```python
from build123d import *

# Parameters (mm, degrees)
F0_R     = 2.6
F1_DEPTH = 2
F2_R     = 2
F3_DEPTH = 25


with BuildPart() as f1:
    # F0 (on Front) → F1 (new body)
    with BuildSketch(Plane.XZ):
        with BuildLine():
            ThreePointArc((-35.5, 0), (0, -35.5), (35.5, 0))
            ThreePointArc((35.5, 0), (0, 35.5), (-35.5, 0))
        make_face()
        with BuildLine():
            ThreePointArc((-18.1, 0), (-20.7, -2.6), (-23.3, 0))
            ThreePointArc((-23.3, 0), (-20.7, 2.6), (-18.1, 0))
        make_face(mode=Mode.SUBTRACT)
        with Locations((20.7, 0)):
            Circle(F0_R, mode=Mode.SUBTRACT)
    extrude(amount=F1_DEPTH)

    # F2 (on face) → F3 (cut)
    with BuildSketch(Plane(origin=(0, 0, 0), x_dir=(-1, 0, 0), z_dir=(0, 1, 0))):
        Circle(F2_R)
        with Locations((0, 7)):
            Circle(F2_R)
        with Locations((0, 14)):
            Circle(F2_R)
        with Locations((0, 21)):
            Circle(F2_R)
        with Locations((0, 28)):
            Circle(F2_R)
        with Locations((7, 0)):
            Circle(F2_R)
        with Locations((7, 7)):
            Circle(F2_R)
        with Locations((7, 14)):
            Circle(F2_R)
        with Locations((7, 21)):
            Circle(F2_R)
        with Locations((7, 28)):
            Circle(F2_R)
        with Locations((14, 0)):
            Circle(F2_R)
        with Locations((14, 7)):
            Circle(F2_R)
        with Locations((14, 14)):
            Circle(F2_R)
        with Locations((14, 21)):
            Circle(F2_R)
        with Locations((14, 28)):
            Circle(F2_R)
        with Locations((21, 7)):
            Circle(F2_R)
        with Locations((21, 14)):
            Circle(F2_R)
        with Locations((21, 21)):
            Circle(F2_R)
        with Locations((28, 0)):
            Circle(F2_R)
        with Locations((28, 7)):
            Circle(F2_R)
        with Locations((28, 14)):
            Circle(F2_R)
        with Locations((-7, 28)):
            Circle(F2_R)
        with Locations((-7, 21)):
            Circle(F2_R)
        with Locations((-7, 14)):
            Circle(F2_R)
        with Locations((-7, 7)):
            Circle(F2_R)
        with Locations((-7, 0)):
            Circle(F2_R)
        with Locations((-14, 28)):
            Circle(F2_R)
        with Locations((-14, 21)):
            Circle(F2_R)
        with Locations((-14, 14)):
            Circle(F2_R)
        with Locations((-14, 7)):
            Circle(F2_R)
        with Locations((-14, 0)):
            Circle(F2_R)
        with Locations((-21, 21)):
            Circle(F2_R)
        with Locations((-21, 14)):
            Circle(F2_R)
        with Locations((-21, 7)):
            Circle(F2_R)
        with Locations((-28, 14)):
            Circle(F2_R)
        with Locations((-28, 7)):
            Circle(F2_R)
        with Locations((-28, 0)):
            Circle(F2_R)
        with Locations((-28, -7)):
            Circle(F2_R)
        with Locations((-21, -7)):
            Circle(F2_R)
        with Locations((-14, -7)):
            Circle(F2_R)
        with Locations((28, -7)):
            Circle(F2_R)
        with Locations((21, -7)):
            Circle(F2_R)
        with Locations((14, -7)):
            Circle(F2_R)
        with Locations((7, -7)):
            Circle(F2_R)
        with Locations((0, -7)):
            Circle(F2_R)
        with Locations((-7, -7)):
            Circle(F2_R)
        with Locations((-28, -14)):
            Circle(F2_R)
        with Locations((-21, -14)):
            Circle(F2_R)
        with Locations((-14, -14)):
            Circle(F2_R)
        with Locations((28, -14)):
            Circle(F2_R)
        with Locations((21, -14)):
            Circle(F2_R)
        with Locations((14, -14)):
            Circle(F2_R)
        with Locations((7, -14)):
            Circle(F2_R)
        with Locations((0, -14)):
            Circle(F2_R)
        with Locations((-7, -14)):
            Circle(F2_R)
        with Locations((-21, -21)):
            Circle(F2_R)
        with Locations((-14, -21)):
            Circle(F2_R)
        with Locations((21, -21)):
            Circle(F2_R)
        with Locations((14, -21)):
            Circle(F2_R)
        with Locations((7, -21)):
            Circle(F2_R)
        with Locations((0, -21)):
            Circle(F2_R)
        with Locations((-7, -21)):
            Circle(F2_R)
        with Locations((-14, -28)):
            Circle(F2_R)
        with Locations((14, -28)):
            Circle(F2_R)
        with Locations((7, -28)):
            Circle(F2_R)
        with Locations((0, -28)):
            Circle(F2_R)
        with Locations((-7, -28)):
            Circle(F2_R)
    extrude(amount=-F3_DEPTH, mode=Mode.SUBTRACT)


solid = f1.part
```
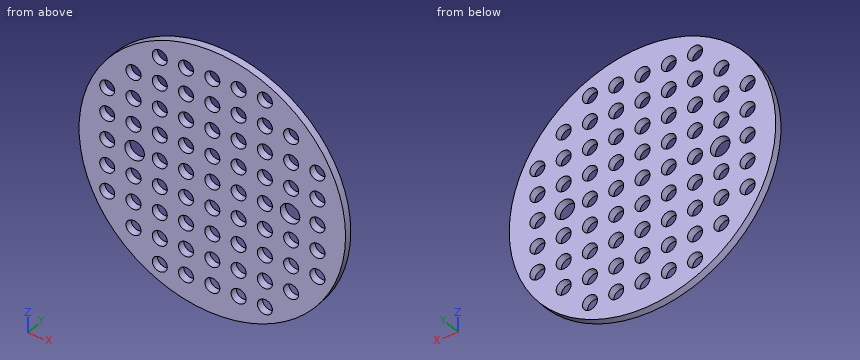
Here's how the part is built. I have some questions about the finished solid (model axes, mm). Round coordinates to 2 decimals unless told otherwise and drop trailing zeros.
1. Suppose I cut it at A-A, the plane x = 0. Give the number of separate pieces and of enclosed holes in the cut face, and give its area (3 significant figures).
Answers:
separate pieces: 10
enclosed holes: 0
area: 70.0 mm2
2. If I drill on probe 1 along Z at (x, y) = (28, -0.55); probe 2 along Z at (x, y) = (2.5, -1.8); probe 3 along X at (y, z) = (-1.15, 3.5), over which ranges is the centre line in solid material (lowest first)?
Answers:
probe 1: z = -21.82 to -16, -12 to -9, -5 to -2, 2 to 5, 9 to 12, 16 to 21.82
probe 2: z = -35.41 to 35.41
probe 3: x = -35.33 to 35.33
3. Will this pin go through, and if not, where does the flat tip stop? pin 1 (2.5 mm diameter, centred on x = 14, z = 7, fed in from +Y).
Answers:
pin 1: passes through
